Source: CAD feature listing. Evaluate the final solid. Frame: model axes, mm. Give positions to 0.01 mm unless a question says otherwise; leave off trailing zeros. Order: outer loops, then holes, each group sorted by start corner. A loop starts at its lowest first (then second) coordinate and runs counter-clockwise, first axis right, second up. Notation, with made-up numbers: (-15, -2.5) - (4, -2.5) arc R24 ccw to (4, 8.5) - close; hole circle Ø8 at (-1.5, -24). An arc over 180 degrees is marked (long way). Answer as CSV lines item,"result".
```python
from build123d import *

# Parameters (mm, degrees)
SKETCH1_R            = 70
BOSS_EXTRUDE1_DEPTH  = 370
SKETCH2_R            = 10
BOSS_EXTRUDE2_DEPTH  = 100
BOSS_EXTRUDE3_START  = 100
SKETCH3_R            = 10
BOSS_EXTRUDE3_DEPTH  = 100
BOSS_EXTRUDE4_START  = -25
BOSS_EXTRUDE4_DEPTH  = 25
BOSS_EXTRUDE5_DEPTH  = 25
SKETCH6_R            = 15
BOSS_EXTRUDE6_DEPTH  = 570
BOSS_EXTRUDE7_START  = 55
SKETCH7_R            = 15
BOSS_EXTRUDE7_DEPTH  = 55
SKETCH8_R            = 15
BOSS_EXTRUDE8_DEPTH  = 55
BOSS_EXTRUDE9_DEPTH  = 55
BOSS_EXTRUDE10_START = -55
BOSS_EXTRUDE10_DEPTH = 55


with BuildPart() as part:
    # Sketch1 → Boss-Extrude1 (new body)
    with BuildSketch(Plane(origin=(0, 0, 0), x_dir=(1, 0, 0), z_dir=(0, 1, 0))):
        with Locations(Location((0, 0, 0), (0, 0, 270))):
            Circle(SKETCH1_R)
    extrude(amount=BOSS_EXTRUDE1_DEPTH)

    # Sketch2 → Boss-Extrude2 (add)
    with BuildSketch(Plane(origin=(0, 370, 0), x_dir=(1, 0, 0), z_dir=(0, 1, 0))):
        with Locations(Location((0, 0, 0), (0, 0, 270))):
            Circle(SKETCH2_R)
    extrude(amount=BOSS_EXTRUDE2_DEPTH)

    # Sketch3 → Boss-Extrude3 (add)
    with BuildSketch(Plane.XZ.offset(BOSS_EXTRUDE3_START)):
        with Locations(Location((0, 0, 0), (0, 0, 90))):
            Circle(SKETCH3_R)
    extrude(amount=-BOSS_EXTRUDE3_DEPTH)

    # Sketch4 → Boss-Extrude4 (add)
    with BuildSketch(Plane(origin=(0, 470, 0), x_dir=(1, 0, 0), z_dir=(0, 1, 0)).offset(BOSS_EXTRUDE4_START)):
        with BuildLine():
            Line((-5, 8.660254038), (-5, 12.820254038))
            Line((-5, 12.820254038), (5, 12.820254038))
            Line((5, 12.820254038), (5, 8.660254038))
            ThreePointArc((5, 8.660254038), (0, 10), (-5, 8.660254038))
        make_face()
    extrude(amount=BOSS_EXTRUDE4_DEPTH)

    # Sketch5 → Boss-Extrude5 (add)
    with BuildSketch(Plane.XZ.offset(100)):
        with BuildLine():
            Line((-5, 8.660254038), (-5, 12.820254038))
            Line((-5, 12.820254038), (5, 12.820254038))
            Line((5, 12.820254038), (5, 8.660254038))
            ThreePointArc((5, 8.660254038), (0, 10), (-5, 8.660254038))
        make_face()
    extrude(amount=-BOSS_EXTRUDE5_DEPTH)

    # Sketch6 → Boss-Extrude6 (add)
    with BuildSketch(Plane.XZ.offset(100)):
        with Locations(Location((0, 0, 0), (0, 0, 270))):
            Circle(SKETCH6_R)
    extrude(amount=-BOSS_EXTRUDE6_DEPTH)

    # Sketch7 → Boss-Extrude7 (add)
    with BuildSketch(Plane.XZ.offset(100).offset(BOSS_EXTRUDE7_START)):
        with Locations(Location((0, 0, 0), (0, 0, 270))):
            Circle(SKETCH7_R)
    extrude(amount=-BOSS_EXTRUDE7_DEPTH)

    # Sketch8 → Boss-Extrude8 (add)
    with BuildSketch(Plane(origin=(0, 470, 0), x_dir=(1, 0, 0), z_dir=(0, 1, 0))):
        with Locations(Location((0, 0, 0), (0, 0, 90))):
            Circle(SKETCH8_R)
    extrude(amount=BOSS_EXTRUDE8_DEPTH)

    # Sketch9 → Boss-Extrude9 (add)
    with BuildSketch(Plane.XZ.offset(155)):
        with BuildLine():
            Line((-5, 14.142135624), (-5, 18.302135624))
            Line((-5, 18.302135624), (5, 18.302135624))
            Line((5, 18.302135624), (5, 14.142135624))
            ThreePointArc((5, 14.142135624), (0, 15), (-5, 14.142135624))
        make_face()
    extrude(amount=-BOSS_EXTRUDE9_DEPTH)

    # Sketch10 → Boss-Extrude10 (add)
    with BuildSketch(Plane(origin=(0, 525, 0), x_dir=(1, 0, 0), z_dir=(0, 1, 0)).offset(BOSS_EXTRUDE10_START)):
        with BuildLine():
            Line((5, -14.142135624), (5, -18.302135624))
            Line((5, -18.302135624), (-5, -18.302135624))
            Line((-5, -18.302135624), (-5, -14.142135624))
            ThreePointArc((-5, -14.142135624), (0, -15), (5, -14.142135624))
        make_face()
    extrude(amount=BOSS_EXTRUDE10_DEPTH)


solid = part.part
```
(1) Cut plane C-C (x = -21). Return loops of the section in (y, z).
Completed:
outline,"(0, -66.78) - (370, -66.78) - (370, 66.78) - (0, 66.78) - close"
(2) Cut plane B-B (y = 386.5). Return loops of the section in (x, z).
Completed:
outline,"circle Ø30 at (0, 0)"
(3) Cut plane A-A (z = 0). Return loops of the section in (x, y), then the cut area to 3 significant figures.
Completed:
outline,"(-70, 0) - (-15, 0) - (-15, -155) - (15, -155) - (15, 0) - (70, 0) - (70, 370) - (15, 370) - (15, 525) - (-15, 525) - (-15, 370) - (-70, 370) - close"
area,"61,100 mm²"
(4) Cut plane D-D (y = 46). Return loops of the section in (x, z).
Completed:
outline,"circle Ø140 at (0, 0)"
(5) Ray query, line 1 (Y direction, x = -8.5, z = 59); line 2 (Z direction, x = -54, y = 15.5). Return the intervals inside material, ascending. Write a range as from..to.
Completed:
line 1,"0..370"
line 2,"-44.54..44.54"
(6) Contact query for flat-ended pins moving along their axis: pin 1 (1.5 mm diameter, centred on x = -30, z = 0.5, fed in from +Y); pin 2 (3 mm diameter, centred on y = 47, z = -9.5, fed in from -X); pin 3 (2 mm diameter, centred on y = 104, z = -12, fed in from -X). Output: stop coordinate, or through.
Completed:
pin 1,"y = 370"
pin 2,"x = -69.54"
pin 3,"x = -69.13"
